Build history of the part. All positions in model axes, mm. Face numbers are marked on the shaded views. A direction names the side the tool comes from. Give positions to 0.01 mm unless a question says otherwise; leave off trailing zeros. Loops run counter-clockwise (first coordinate to the right, second up) from the corner with the lowest first, then second, coordinate; pieces in that order, holes last.
1) Flat gauge pins, fed straight in: P1, Ø4, axis at y = 5.5, z = 51.5, coming from the +X side; P2, Ø6, axis at x = -24, y = -7.5, coming from the +Z side. Where does each tip first touch, or does it go through?
2) Band-saw the part on C-C on x = 10. List the corners of the cut face in (y, z), then the cut area to 3 significant figures.
3) Band-saw the part on A-A on z = 58.5. List the corners of the cut face in (x, y), then the cut area to 3 significant figures.
4) Wall check: line 1 (X direction, y = 14.5, z = 39); line 2 (Z direction, x = 1.5, y = 22); line 3 (Y direction, x = -40, z = 69.5). Give the ranges that are in metal, low to high.
5) 3-axis set-ups, long thin cutter, end or side, ignore diameter. For the marked faces 1 and 2: which of +Z, -Z, +X, -X, +Y, -Y reach the whole face in a straight line?
6) Band-saw the part on D-D on z = 49. List the corners of the cut face in (x, y).
7) Band-saw the part on B-B on y = -20. List the corners of the cut face in (x, z), then the cut area to 3 significant figures.
8) Two-plate mould, pull along Y, no slides. Class the marked faces 3, 4, 5 and 6: +Y half, -Y half, draft (parallel to the pull), parting line (faces both ways), or undercut.
```python
from build123d import *

# Parameters (mm, degrees)
F0_W     = 92.3780202866
F0_H     = 63.4378064424
F1_DEPTH = 25.4
F2_W     = 38.2190011442
F2_H     = 63.4378064424
F3_DEPTH = 50.8
F7_DEPTH = 50.8


# Not quite as in the source:
# - the program builds the solid bodies; features that only make, move or delete a surface that nothing else refers to are left out


with BuildPart() as f1:
    # F0 (on Top) → F1 (new body)
    with BuildSketch(Plane.XY):
        with Locations((-0.0018253922, 5.7058585808)):
            Rectangle(F0_W, F0_H)
    extrude(amount=F1_DEPTH)

    # F2 (on face) → F3 (join)
    with BuildSketch(Plane.XY.offset(25.4)):
        with Locations((-27.0813349634, 5.7058585808)):
            Rectangle(F2_W, F2_H)
    extrude(amount=F3_DEPTH)

    # F6 (on face) → F7 (cut)
    with BuildSketch(Plane.YZ.offset(-7.9718343914)):
        with BuildLine():
            ThreePointArc((-17.3291587886, 76.2), (5.7058585808, 53.1649826306), (28.7408759501, 76.2))
            Line((28.7408759501, 76.2), (-17.3291587886, 76.2))
        make_face()
    extrude(amount=-F7_DEPTH, mode=Mode.SUBTRACT)


solid = f1.part
```
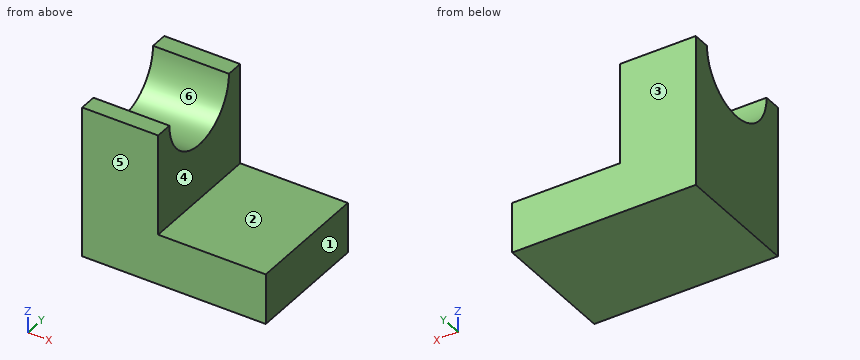
Findings below:
1. P1: stops at x = -7.97
1. P2: stops at z = 59.83
2. outline: (-26.01, 0) - (37.42, 0) - (37.42, 25.4) - (-26.01, 25.4) - close
2. area: 1,610 mm2
3. outline: (-46.19, -26.01) - (-7.97, -26.01) - (-7.97, -9.04) - (-46.19, -9.04) - close; (-46.19, 20.45) - (-7.97, 20.45) - (-7.97, 37.42) - (-46.19, 37.42) - close
3. area: 1,300 mm2
4. line 1: x = -46.19 to -7.97
4. line 2: z = 0 to 25.4
4. line 3: y = -26.01 to -16.33, 27.74 to 37.42
5. face 1: +Z, -Z, +X, +Y, -Y
5. face 2: +Z, +X, +Y, -Y
6. outline: (-46.19, -26.01) - (-7.97, -26.01) - (-7.97, 37.42) - (-46.19, 37.42) - close
7. outline: (-46.19, 0) - (46.19, 0) - (46.19, 25.4) - (-7.97, 25.4) - (-7.97, 76.2) - (-46.19, 76.2) - close
7. area: 4,290 mm2
8. face 3: +Y half
8. face 4: draft
8. face 5: -Y half
8. face 6: undercut
